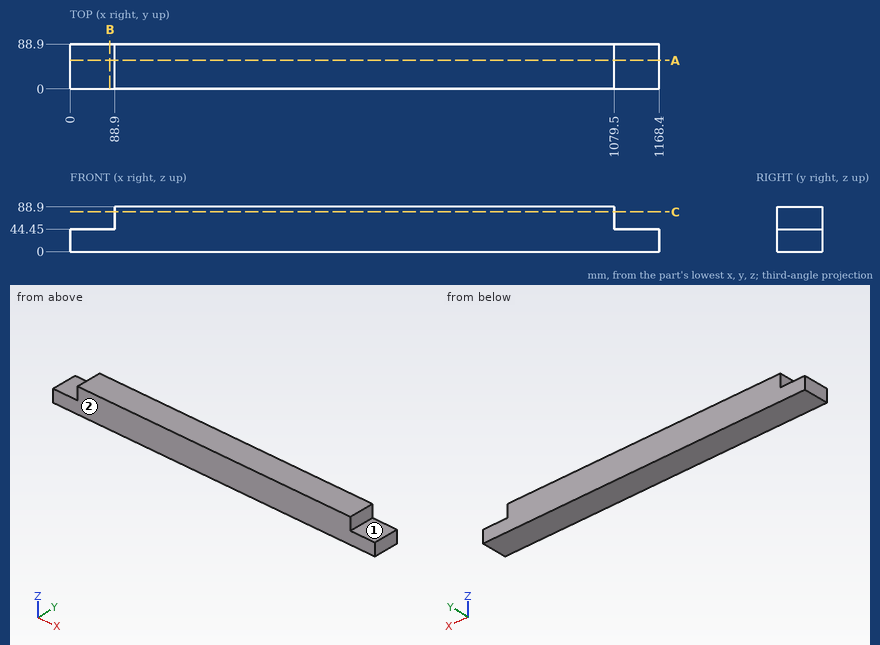
Geometry: see drawing. Coordinates: mm, zero at the bounding-box minimum. A direction names the side the tool comes from. Coordinates: 2 decimals unless noted, no trailing zeros. Loops run counter-clockwise (first coordinate to the right, second up) from the corner with the lowest first, then second, coordinate; pieces in that order, holes last.
(1) Section B-B on x = 79. Return the cut outline in (y, z).
(2) Set-up query: the marked faces 1 and 2. Return all of +Z, -Z, +X, -X, +Y, -Y with unobstructed straight access to the full face (end or side cutting, diameter ignored); none if empty.
(3) First-contact query: pin 1 Ø5 at (y, z) = (65.5, 74) entering from -X; pin 2 Ø1.5 at (y, z) = (79.5, 52.5) entering from +X. Flat tips, straight axial feed; report the tip coordinate or a pass-through.
(4) Section A-A on y = 56.5. Return the cut outline in (x, z), then the cut area to 3 significant figures.
(5) Section C-C on z = 79. Return the cut outline in (x, y), then the cut area to 3 significant figures.
(6) Material intervals for probe 1 along X at (y, z) = (31.5, 64.5); probe 2 along Z at (x, y) = (59, 58), sorted ascending.
Data:
1. outline: (0, 0) - (88.9, 0) - (88.9, 44.45) - (0, 44.45) - close
2. face 1: +Z, +X, +Y, -Y
2. face 2: +Z, -Z, +X, -X, -Y
3. pin 1: stops at x = 88.9
3. pin 2: stops at x = 1079.5
4. outline: (0, 0) - (1168.4, 0) - (1168.4, 44.45) - (1079.5, 44.45) - (1079.5, 88.9) - (88.9, 88.9) - (88.9, 44.45) - (0, 44.45) - close
4. area: 96,000 mm2
5. outline: (88.9, 0) - (1079.5, 0) - (1079.5, 88.9) - (88.9, 88.9) - close
5. area: 88,100 mm2
6. probe 1: x = 88.9 to 1079.5
6. probe 2: z = 0 to 44.45
